Input: part model. Units: mm. Frame: model coordinates. Give positions to 0.01 mm unless a question says otherwise; leave off trailing zeros. Loops run counter-clockwise (first coordinate to the right, second up) from the corner with the lowest first, then second, coordinate; pieces in that order, holes last. Notation, with made-up numbers: M -29,47 L -25,47 A10 ccw -25,53 Z; hole C 86.5,39 d3. An arc over 180 degrees is marked long. Answer as a JSON object with one key per item and string values. Group by question number.
1) Section query A-A on x = -74.25. Return loops of the section in (y, z).
2) First-contact query: P1, Ø1.2, axis at x = -77, y = -28, coming from the -Z side; P2, Ø0.8, axis at y = -28, z = -0.5, coming from the +X side; P3, Ø0.7, axis at y = -29, z = 0.5, coming from the -X side; P4, Ø0.7, axis at y = -29.5, z = 0.5, coming from the -X side. Flat tips, straight axial feed; report the tip coordinate or a pass-through.
3) Ray query, L1, parallel to Y at x = -76, z = 0.15; L2, parallel to Z at x = -79.25, y = -30.1; L3, parallel to X at y = -28.7, z = 0.55. Return the intervals inside material, ascending.
4) Section query B-B on z = -0.4. Return loops of the section in (x, y).
5) Section query C-C on x = -71.5. Return loops of the section in (y, z).
from build123d import *

# Parameters (mm, degrees)
CROQUIS1_W              = 4.5
CROQUIS1_H              = 3.47922044
SALIENTE_EXTRUIR1_DEPTH = 0.6
REDONDEO1_R             = 0.5
CROQUIS2_W              = 0.3
CROQUIS2_H              = 0.738230838
SALIENTE_EXTRUIR2_DEPTH = 0.8


with BuildPart() as part:
    # Croquis1 → Saliente-Extruir1 (new body)
    with BuildSketch(Plane.XY):
        with BuildLine():
            Line((-80.458731062, -26.409325636), (-69.586167188, -26.409325636))
            add(Edge.make_bspline(
                [(-69.586167188, -26.409325636), (-67.825300142, -26.409325636), (-66.171601872, -28.063804878), (-65.9618826, -30.409325636)],
                knots=[0, 0, 0, 0, 1, 1, 1, 1], degree=3))
            Line((-65.9618826, -30.409325636), (-69.586167188, -30.409325636))
            Line((-69.586167188, -30.409325636), (-80.458731062, -30.409325636))
            Line((-80.458731062, -30.409325636), (-80.458731062, -28.778441055))
            Line((-80.458731062, -28.778441055), (-81.328536172, -28.778441055))
            Line((-81.328536172, -28.778441055), (-81.328536172, -28.040210217))
            Line((-81.328536172, -28.040210217), (-80.458731062, -28.040210217))
            Line((-80.458731062, -28.040210217), (-80.458731062, -26.409325636))
        make_face()
        with Locations((-75.022449125, -28.409325636)):
            Rectangle(CROQUIS1_W, CROQUIS1_H, mode=Mode.SUBTRACT)
    extrude(amount=SALIENTE_EXTRUIR1_DEPTH)

    # Redondeo1
    redondeo1_edges = [part.edges().sort_by_distance(p)[0] for p in [
        (-77.272449125, -26.669715416, 0.3),
        (-77.272449125, -30.148935856, 0.3),
        (-72.772449125, -30.148935856, 0.3),
        (-72.772449125, -26.669715416, 0.3),
    ]]
    fillet(redondeo1_edges, radius=REDONDEO1_R)

    # Croquis2 → Saliente-Extruir2 (add)
    with BuildSketch(Plane(origin=(0, 0, 0), x_dir=(-1, 0, 0), z_dir=(0, 0, -1))):
        with Locations((81.178536172, -28.409325636)):
            Rectangle(CROQUIS2_W, CROQUIS2_H)
    extrude(amount=SALIENTE_EXTRUIR2_DEPTH)


solid = part.part
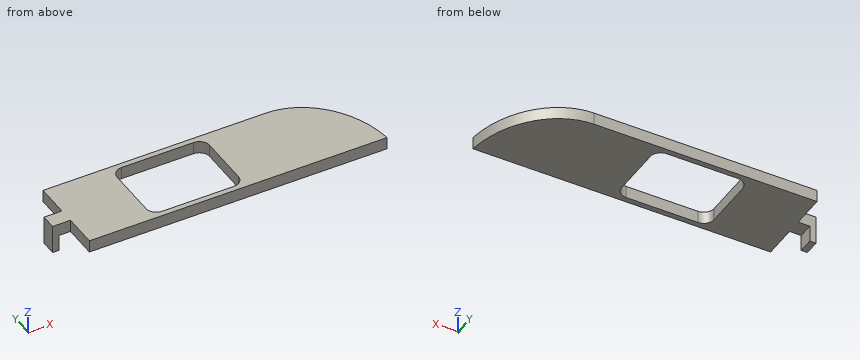
Output:
{
 "1": {"outline": "M -30.41,0 L -30.15,0 L -30.15,0.6 L -30.41,0.6 Z; M -26.67,0 L -26.41,0 L -26.41,0.6 L -26.67,0.6 Z"},
 "2": {"P1": "stops at z = 0", "P2": "stops at x = -81.03", "P3": "stops at x = -81.33", "P4": "stops at x = -80.46"},
 "3": {"L1": "y = -30.41 to -30.15, -26.67 to -26.41", "L2": "z = 0 to 0.6", "L3": "x = -81.33 to -77.27, -72.77 to -66.41"},
 "4": {"outline": "M -81.33,-28.78 L -81.03,-28.78 L -81.03,-28.04 L -81.33,-28.04 Z"},
 "5": {"outline": "M -30.41,0 L -26.41,0 L -26.41,0.6 L -30.41,0.6 Z"}
}
